Input: part model. Units: mm. Frame: model coordinates. A direction names the side the tool comes from. Round coordinates to 2 decimals unless told otherwise and drop trailing zeros. Loops run counter-clockwise (first coordinate to the right, second up) from the corner with the lowest first, then second, coordinate; pieces in that order, holes last.
(1) Draft query along Z for faces 1 (the face through (22.14, 13.306, 7.262)), 2 (the face through (23.709, 14.236, -5.472)), 3 (the face through (-2, 2, 4)). Return one class per face: released by +Z, released by -Z, zero draft, split by the parting line, or undercut.
(2) Cut plane B-B, the plane y = 0. Output: boundary loops of the cut face in (x, z), and give its area (3 significant figures).
(3) Cut plane C-C, the plane x = 1. Output: boundary loops of the cut face in (y, z), and give its area (3 significant figures).
(4) First-contact query: pin 1 Ø1.5 at (y, z) = (5.5, -1.5) entering from -X; pin 2 Ø0.8 at (x, y) = (26, 15.5) entering from -Z; pin 3 Ø5 at (x, z) = (21, 1) entering from -Y. Flat tips, straight axial feed; report the tip coordinate or a pass-through.
(5) Cut plane D-D, the plane x = 12.5. Output: boundary loops of the cut face in (y, z), and give its area (3 significant figures).
(6) Line query: line 1 (X direction, y = 12.25, z = 5.5); line 2 (X direction, y = 12.75, z = -4.75); line 3 (X direction, y = -0.5, z = -1.25). Output: solid intervals per line, ascending.
(7) Access query for faces 4 (the face through (7.759, 7.802, 0.021)), 5 (the face through (23, 17, -6)), 6 (the face through (25, 16.5, 5.5)). Directions: +Z, -Z, +X, -X, +Y, -Y. A direction counts if a zero-diameter tool reaches every point of the face in a straight line with its end or side. Return the directions, or none.
from build123d import *

# Parameters (mm, degrees)
CROQUIS1_R              = 3.96875
SALIENTE_EXTRUIR1_DEPTH = 7.5
CROQUIS2_W              = 2.5
CROQUIS2_H              = 3.96875
CORTAR_EXTRUIR1_DEPTH   = 15
CROQUIS4_R              = 2.38125
CORTAR_EXTRUIR2_DEPTH   = 15
CROQUIS5_R              = 5.55625
CORTAR_EXTRUIR3_DEPTH   = 5
CROQUIS8_W              = 1
CROQUIS8_H              = 1.5
CORTAR_EXTRUIR6_DEPTH   = 4
CROQUIS10_R             = 4
CROQUIS10_R_2           = 1.5
CORTAR_EXTRUIR7_DEPTH   = 1.5


with BuildPart() as part:
    # Croquis1 → Saliente-Extruir1 (new, symmetric)
    with BuildSketch(Plane.XY):
        Circle(CROQUIS1_R)
        with BuildLine():
            Line((13.356089924, 18.96875), (-2.806330038, 2.806330038))
            ThreePointArc((-2.806330038, 2.806330038), (1.518774872, 3.666646895), (3.96875, 0))
            ThreePointArc((3.96875, 0), (3.666646895, -1.518774872), (2.806330038, -2.806330038))
            Line((2.806330038, -2.806330038), (16.643910076, 11.03125))
            Line((16.643910076, 11.03125), (25, 11.03125))
            ThreePointArc((25, 11.03125), (21.03125, 15), (25, 18.96875))
            Line((25, 18.96875), (13.356089924, 18.96875))
        make_face()
        with BuildLine():
            ThreePointArc((28.96875, 15), (27.806330038, 17.806330038), (25, 18.96875))
            Line((25, 18.96875), (25, 11.03125))
            ThreePointArc((25, 11.03125), (27.806330038, 12.193669962), (28.96875, 15))
        make_face()
        with BuildLine():
            Line((25, 11.03125), (25, 18.96875))
            ThreePointArc((25, 18.96875), (21.03125, 15), (25, 11.03125))
        make_face()
        with BuildLine():
            ThreePointArc((28.96875, 15), (27.806330038, 17.806330038), (25, 18.96875))
            Line((25, 18.96875), (25, 11.03125))
            ThreePointArc((25, 11.03125), (27.806330038, 12.193669962), (28.96875, 15))
        make_face()
        with BuildLine():
            Line((25, 11.03125), (25, 18.96875))
            ThreePointArc((25, 18.96875), (21.03125, 15), (25, 11.03125))
        make_face()
    extrude(amount=SALIENTE_EXTRUIR1_DEPTH, both=True)

    # Croquis2 → Cortar-Extruir1 (cut)
    with BuildSketch(Plane(origin=(-2.806330038, 2.806330038, 0), x_dir=(0, 0, 1), z_dir=(-0.7071067811865441, 0.7071067811865509, 0))):
        with Locations((-3.75, -1.984375)):
            Rectangle(CROQUIS2_W, CROQUIS2_H)
        with Locations((3.75, -1.984375)):
            Rectangle(CROQUIS2_W, CROQUIS2_H)
    extrude(amount=-CORTAR_EXTRUIR1_DEPTH, mode=Mode.SUBTRACT)

    # Croquis4 → Cortar-Extruir2 (cut)
    with BuildSketch(Plane.XY.offset(7.5)):
        Circle(CROQUIS4_R)
    extrude(amount=-CORTAR_EXTRUIR2_DEPTH, mode=Mode.SUBTRACT)

    # Croquis5 → Cortar-Extruir3 (cut)
    with BuildSketch(Plane.XY.offset(7.5)):
        with Locations((25, 15)):
            Circle(CROQUIS5_R)
    cortar_extruir3 = extrude(amount=-CORTAR_EXTRUIR3_DEPTH, mode=Mode.SUBTRACT)

    # Simetría1: Cortar-Extruir3 across plane
    add(cortar_extruir3.mirror(Plane.XY), mode=Mode.SUBTRACT)

    # Croquis8 → Revolución1 (revolve)
    with BuildSketch(Plane(origin=(25, 0, 0), x_dir=(0, 0, -1), z_dir=(1, 0, 0)), mode=Mode.PRIVATE) as revoluci_n1_sk:
        Polygon((7.5, 18.175), (7.5, 16.5), (2.5, 16.5), (2.5, 18.175), (6.441294167, 18.175), (6.62, 18.725), align=None)
        with Locations((3, 15.75)):
            Rectangle(CROQUIS8_W, CROQUIS8_H)
    revoluci_n1 = revolve(revoluci_n1_sk.sketch.rotate(Axis((25, 15, -2.5), (0, 0, -1)), 90), axis=Axis((25, 15, -2.5), (0, 0, -1)))

    # Croquis9 → Cortar-Extruir6 (cut)
    with BuildSketch(Plane(origin=(0, 0, -7.5), x_dir=(-1, 0, 0), z_dir=(0, 0, -1))):
        with BuildLine():
            Line((-23.777080012, 10.436000471), (-25, 15))
            Line((-25, 15), (-26.222919988, 10.436000471))
            ThreePointArc((-26.222919988, 10.436000471), (-25, 10.275), (-23.777080012, 10.436000471))
        make_face()
        with BuildLine():
            Line((-29.563999529, 16.222919988), (-25, 15))
            Line((-25, 15), (-28.341079541, 18.341079541))
            ThreePointArc((-28.341079541, 18.341079541), (-29.091970033, 17.3625), (-29.563999529, 16.222919988))
        make_face()
        with BuildLine():
            Line((-21.658920459, 18.341079541), (-25, 15))
            Line((-25, 15), (-20.436000471, 16.222919988))
            ThreePointArc((-20.436000471, 16.222919988), (-20.908029967, 17.3625), (-21.658920459, 18.341079541))
        make_face()
    cortar_extruir6 = extrude(amount=-CORTAR_EXTRUIR6_DEPTH, mode=Mode.SUBTRACT)

    # Simetría2: Revolución1, Cortar-Extruir6 across plane
    add(revoluci_n1.mirror(Plane.XY))
    add(cortar_extruir6.mirror(Plane.XY), mode=Mode.SUBTRACT)

    # Croquis10 → Cortar-Extruir7 (cut, symmetric)
    with BuildSketch(Plane.XY):
        with Locations((10.52444577, 4.911785694)):
            Circle(CROQUIS10_R)
        with Locations((10.52444577, 4.911785694)):
            Circle(CROQUIS10_R_2, mode=Mode.SUBTRACT)
    extrude(amount=CORTAR_EXTRUIR7_DEPTH, both=True, mode=Mode.SUBTRACT)


solid = part.part
Reported:
1. face 1: released by +Z
1. face 2: zero draft
1. face 3: undercut
2. outline: (-3.97, -7.5) - (-2.38, -7.5) - (-2.38, -5) - (-3.97, -5) - close; (-3.97, -2.5) - (-2.38, -2.5) - (-2.38, 2.5) - (-3.97, 2.5) - close; (-3.97, 5) - (-2.38, 5) - (-2.38, 7.5) - (-3.97, 7.5) - close; (2.38, -7.5) - (5.61, -7.5) - (5.61, 7.5) - (2.38, 7.5) - close
2. area: 64.3 mm2
3. outline: (-3.84, -7.5) - (-2.16, -7.5) - (-2.16, -5) - (-3.84, -5) - close; (-3.84, -2.5) - (-2.16, -2.5) - (-2.16, 2.5) - (-3.84, 2.5) - close; (-3.84, 5) - (-2.16, 5) - (-2.16, 7.5) - (-3.84, 7.5) - close; (2.16, -7.5) - (6.61, -7.5) - (6.61, 7.5) - (2.16, 7.5) - close
3. area: 83.6 mm2
4. pin 1: stops at x = -0.86
4. pin 2: stops at z = -3.5
4. pin 3: stops at y = 11.03
5. outline: (6.89, -7.5) - (18.11, -7.5) - (18.11, 7.5) - (6.89, 7.5) - (6.89, 1.5) - (8.39, 1.5) - (8.39, -1.5) - (6.89, -1.5) - close
5. area: 164 mm2
6. line 1: x = 6.64 to 20.17, 23.41 to 24.26, 25.74 to 26.59
6. line 2: x = 7.14 to 19.92, 22.76 to 24.4, 25.6 to 27.24
6. line 3: x = -3.94 to -2.33, 2.33 to 5.11
7. face 4: none
7. face 5: -Z
7. face 6: +Z
